Design review of the part built by this model. Coordinates are the model's own, in mm. Face numbers are marked on the shaded views. Give positions to 0.01 mm unless a question says otherwise; leave off trailing zeros. Write each loop counter-clockwise with the first axis right and the second up, starting at its lowest first coordinate (ties: lowest second). Pieces come first, ordered by that corner, then holes. Notation, with made-up numbers: M 70.25,-39.75 L 94.25,-39.75 A22 cw 94.25,-25.75 Z; hole C 75.25,-30.5 d4. An arc over 180 degrees is marked long. Write each question's results on one line, items separated by ' | '. Start each with the question number.
from build123d import *

# Parameters (mm, degrees)
SKETCH1_W              = 30
SKETCH1_H              = 30
BOSS_EXTRUDE1_DEPTH    = 6.35
F_2_CLEARANCE_HOLE1_D  = 2.2606
SKETCH4_R              = 4.99999
CUT_EXTRUDE1_DEPTH     = 43.898980174
M2_5_CLEARANCE_HOLE1_D = 2.7
SKETCH9_R              = 0.9779
CUT_EXTRUDE2_DEPTH     = 43.898980174


with BuildPart() as part:
    # Sketch1 → Boss-Extrude1 (new body)
    with BuildSketch(Plane.XY):
        with Locations((15, 15)):
            Rectangle(SKETCH1_W, SKETCH1_H)
    extrude(amount=BOSS_EXTRUDE1_DEPTH)

    # #2 Clearance Hole1 (through all)
    with Locations(Plane.XY.offset(6.35)):
        with Locations((2.5, 27.5), (27.5, 27.5), (2.5, 2.5), (27.5, 2.5)):
            Hole(F_2_CLEARANCE_HOLE1_D / 2)

    # Sketch4 → Cut-Extrude1 (cut, through all)
    with BuildSketch(Plane.XY.offset(6.35)):
        with Locations((12.55014, 15.00124)):
            Circle(SKETCH4_R)
    extrude(amount=-CUT_EXTRUDE1_DEPTH, mode=Mode.SUBTRACT)

    # M2.5 Clearance Hole1 (through all)
    with Locations(Plane.XY.offset(6.35)):
        with Locations((16.551324598, 8.072566042), (8.550324637, 8.071775514), (4.549140039, 15.000449472), (8.548955402, 21.929913958), (16.549955363, 21.930704486)):
            Hole(M2_5_CLEARANCE_HOLE1_D / 2)

    # Sketch9 → Cut-Extrude2 (cut, through all)
    with BuildSketch(Plane.XY.offset(6.35)):
        with Locations((22.40032, 15)):
            Circle(SKETCH9_R)
    extrude(amount=-CUT_EXTRUDE2_DEPTH, mode=Mode.SUBTRACT)


solid = part.part
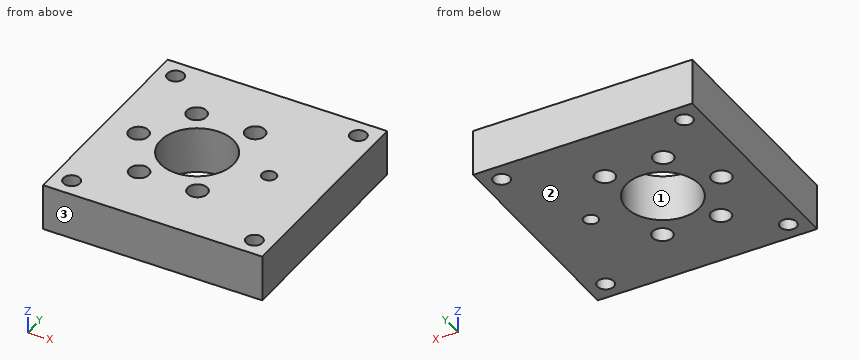
Q1. Wall thickness on line 1 along Y through (x, z) = (27.5, 2); line 2 along X through (y, z) = (22, 5.5); line 3 along Y through (x, z) = (22.5, 1.25): over which ranges is each line inside the solid? List them lowest first. Write a range as from..to.
Q2. We need section A-A on y = 27.5. Write out the cut boundary in (x, z), and give its area (3 significant figures).
Q3. The part is to be moulded in two halves that separate along Y. For the marked faces 1, 2 and 3, say which applies: pulls with the +Y half, pulls with the -Y half, needs draft (parallel to the pull), parting line crosses it, or undercut.
Q4. We need section C-C on z = 5.25. Count the separate pieces of the cut face and the enclosed holes in it, and give its area (3 significant figures).
Q5. For pin 1 Ø1.6 at (x, y) = (22.4, 15) entering from -Z; pin 2 Ø2 at (y, z) = (6.5, 2.5) entering from -X, all flat-tipped, find the tip position at first contact; note any pin that passes through.
Answer sheet:
1) line 1: 0..1.37, 3.63..26.37, 28.63..30 | line 2: 0..7.2, 9.9..15.2, 17.9..30 | line 3: 0..14.03, 15.97..30
2) outline: M 0,0 L 1.37,0 L 1.37,6.35 L 0,6.35 Z; M 3.63,0 L 26.37,0 L 26.37,6.35 L 3.63,6.35 Z; M 28.63,0 L 30,0 L 30,6.35 L 28.63,6.35 Z | area: 162 mm^2
3) face 1: undercut | face 2: needs draft | face 3: pulls with the -Y half
4) separate pieces: 1 | enclosed holes: 11 | area: 774 mm^2
5) pin 1: through | pin 2: x = 0
